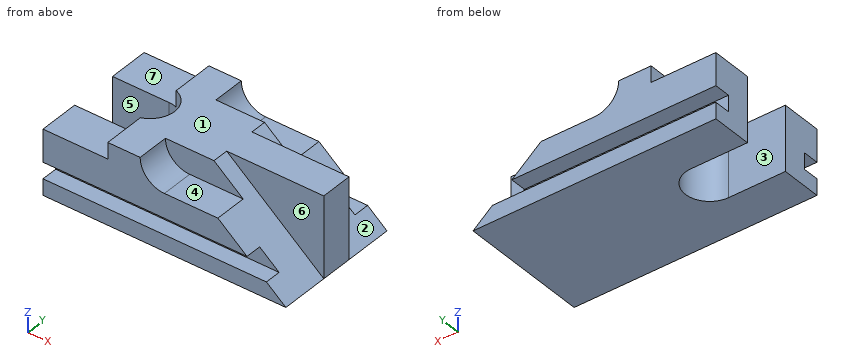
```python
from build123d import *

# Parameters (mm, degrees)
F1_DEPTH = 50
F2_W     = 40
F2_H     = 10
F3_DEPTH = 30
F4_DEPTH = 10
F5_DEPTH = 20


# Not quite as in the source:
# - a pattern or mirror of a feature is missing from the dataset's text; its kind, count and spacing are read off the source's solid


with BuildPart() as f1:
    # F0 (on Top) → F1 (new body)
    with BuildSketch(Plane.XY):
        with BuildLine():
            Line((-35, -15), (-35, -40))
            Line((-35, -40), (115, -40))
            Line((115, -40), (115, 40))
            Line((115, 40), (-35, 40))
            Line((-35, 40), (-35, 15))
            Line((-35, 15), (0, 15))
            ThreePointArc((0, 15), (15, 0), (0, -15))
            Line((0, -15), (-35, -15))
        make_face()
    extrude(amount=F1_DEPTH)

    # F2 (on face) → F3 (cut)
    with BuildSketch(Plane.XZ.offset(40)):
        with Locations((-15, 45)):
            Rectangle(F2_W, F2_H)
        Polygon((115, 50), (55, 50), (73, 35), (91, 20), (103, 10), (115, 0), align=None)
    f3 = extrude(amount=-F3_DEPTH, mode=Mode.SUBTRACT)

    # F3_copies: F3 across plane
    add(f3.mirror(Plane.ZX), mode=Mode.SUBTRACT)

    # F2 (on face) → F4 (cut)
    with BuildSketch(Plane.XZ.offset(40)):
        Polygon((91, 20), (-35, 20), (-35, 10), (103, 10), align=None)
    f4 = extrude(amount=-F4_DEPTH, mode=Mode.SUBTRACT)

    # F4_copies: F4 across plane
    add(f4.mirror(Plane.ZX), mode=Mode.SUBTRACT)

    # F2 (on face) → F5 (cut)
    with BuildSketch(Plane.XZ.offset(40)):
        with BuildLine():
            Line((55, 50), (25, 50))
            ThreePointArc((25, 50), (29.3933982822, 39.3933982822), (40, 35))
            Line((40, 35), (73, 35))
            Line((73, 35), (55, 50))
        make_face()
    f5 = extrude(amount=-F5_DEPTH, mode=Mode.SUBTRACT)

    # F5_copies: F5 across plane
    add(f5.mirror(Plane.ZX), mode=Mode.SUBTRACT)


solid = f1.part
```
Geometry check sheet. Reference: the model listing, model coordinates, mm. Face numbers are marked on the shaded views. A direction names the side the tool comes from. Round coordinates to 2 decimals unless told otherwise and drop trailing zeros. Loops run counter-clockwise (first coordinate to the right, second up) from the corner with the lowest first, then second, coordinate; pieces in that order, holes last. Notation, with made-up numbers: (74, -30) - (98, -30) arc R27 ccw to (98, -3) - close; hole circle Ø6 at (44.25, 64.5). An arc over 180 degrees is marked (long way). Write item = value, one per line. Start each with the question number.
1. Section check A-A on x = -21. Enter the section's corners in (y, z).
2. Section check D-D on y = -27. Enter the section's corners in (x, z).
3. Set-up check for the marked faces 1, 2, 3 and 4: record each of +Z, -Z, +X, -X, +Y, -Y from which the full face is reachable in a straight line by a thin tool's end or side.
4. Depth check by flat-ended pin: pin 1 (8 mm diameter, centred on x = 58, z = 44, fed in from -Y); pin 2 (13 mm diameter, centred on x = -13.5, y = -21, fed in from +Z); pin 3 (1 mm diameter, centred on y = 9, z = 32, fed in from -X). Enter the tip coordinate at first touch or a pass-through.
5. Section check C-C on z = 22.5. Enter the section's corners in (x, y).
6. Section check B-B on y = 35. Enter the section's corners in (x, z), then the cut area to 3 significant figures.
7. Thickness scan on line 1 (Z direction, x = 47, y = 34.5); line 2 (Y direction, x = -18, z = 9); line 3 (Z direction, x = 1.5, y = 32). Record the ranges inside material, lowest first.
8. Mould release check, pull along Y, two halves, no side actions. Record for the marked faces 5, 6 and 7: released by +Y, released by -Y, zero draft, split by the parting line, or undercut.
Working result:
q1.outline = (-40, 0) - (-15, 0) - (-15, 40) - (-40, 40) - (-40, 20) - (-30, 20) - (-30, 10) - (-40, 10) - close; (15, 0) - (40, 0) - (40, 10) - (30, 10) - (30, 20) - (40, 20) - (40, 40) - (15, 40) - close
q2.outline = (-35, 0) - (115, 0) - (73, 35) - (40, 35) arc R15 cw to (25, 50) - (5, 50) - (5, 40) - (-35, 40) - close
q3.face_1 = +Z, +X, -X, +Y, -Y
q3.face_2 = +Z, +X, +Y
q3.face_3 = +Z, -Z, -X
q3.face_4 = +Z, +X, -Y
q4.pin_1 = -20
q4.pin_2 = 40
q4.pin_3 = 11.61
q5.outline = (-35, -40) - (88, -40) - (88, -10) - (115, -10) - (115, 10) - (88, 10) - (88, 40) - (-35, 40) - (-35, 15) - (0, 15) arc R15 cw to (0, -15) - (-35, -15) - close
q6.outline = (-35, 0) - (115, 0) - (103, 10) - (-35, 10) - close; (-35, 20) - (91, 20) - (73, 35) - (40, 35) arc R15 cw to (25, 50) - (5, 50) - (5, 40) - (-35, 40) - close
q6.area = 3,740 mm^2
q7.line_1 = 0 to 10, 20 to 35
q7.line_2 = -40 to -15, 15 to 40
q7.line_3 = 0 to 10, 20 to 40
q8.face_5 = undercut
q8.face_6 = released by -Y
q8.face_7 = zero draft
